Here's how the part is built. I have some questions about the finished solid (model axes, mm). A direction names the side the tool comes from. Round coordinates to 2 decimals unless told otherwise and drop trailing zeros. Order: outer loops, then holes, each group sorted by start corner. A loop starts at its lowest first (then second) coordinate and runs counter-clockwise, first axis right, second up. Notation, with made-up numbers: M 5,34 L 51,34 A8 cw 51,45 Z; hole C 81.25,-26.5 d7. An arc over 180 degrees is marked long. Write item = value, one per line. Start each with the question number.
Item 1: For faces 4 (the face through (1.53, 10.19, 2.95)), 5 (the face through (-0.22, 6.1, -1.71)), which set-ups out of +Z, -Z, +X, -X, +Y, -Y let a thin tool reach every point of the face, with its end or its side?
Item 2: Please list where these lines run through material, in increasing order: L1, parallel to Y at x = -2, z = 0; L2, parallel to Y at x = -1.5, z = 0.25; L3, parallel to X at y = 4.5, z = -1.5.
Item 3: I want a section at A-A, the plane y = 6.5. List the corners of the cut face in (x, z) for me (3 decimals).
Item 4: We'd pull the mould along X, two halves only. Please class faces 1 (the face through (0, 11.1, 0)), 2 (the face through (0.304, 1.141, 0.584)), 3 (the face through (1.35, 9.3, 1.35)): pulls with the +X half, pulls with the -X half, needs draft (parallel to the pull), parting line crosses it, or undercut.
Item 5: I'm going to push flat-ended pins straight in: P1, Ø3, axis at x = -1, y = 5, coming from the -Z side (3 decimals); P2, Ø3, axis at x = -0.5, z = 2, coming from the -Y side; P3, Ø1.5, axis at x = 2.5, y = 10.5, coming from the -Z side. Where does each tip first touch, or does it pass through?
Item 6: I want a section at B-B, the plane y = 2. List the corners of the cut face in (x, z) for me.
```python
from build123d import *

# Parameters (mm, degrees)
CORTAR_EXTRUIR1_START = -1.8
CORTAR_EXTRUIR1_DEPTH = 3


with BuildPart() as part:
    # Croquis1 → Revolución1 (revolve)
    with BuildSketch(Plane.XY):
        with BuildLine():
            Line((0, 0), (0, 11.8))
            ThreePointArc((0, 11.8), (1.722325826, 11.57102319), (3.325, 10.9))
            Line((3.325, 10.9), (3.325, 9.5))
            ThreePointArc((3.325, 9.5), (3.266421356, 9.358578644), (3.125, 9.3))
            Line((3.125, 9.3), (1.725, 9.3))
            Line((1.725, 9.3), (1.725, 2.987787643))
            Line((1.725, 2.987787643), (0, 0))
        make_face()
    revolve(axis=Axis((0, 0, 0), (0, 1, 0)))

    # Croquis2 → Cortar-Extruir1 (cut)
    with BuildSketch(Plane.XZ.offset(-9.3).offset(CORTAR_EXTRUIR1_START)):
        with BuildLine():
            Line((-0.4, 3.2), (-0.4, 0.9))
            ThreePointArc((-0.4, 0.9), (-0.546446609, 0.546446609), (-0.9, 0.4))
            Line((-0.9, 0.4), (-3.2, 0.4))
            Line((-3.2, 0.4), (-3.2, -0.4))
            Line((-3.2, -0.4), (-0.9, -0.4))
            ThreePointArc((-0.9, -0.4), (-0.546446609, -0.546446609), (-0.4, -0.9))
            Line((-0.4, -0.9), (-0.4, -3.2))
            Line((-0.4, -3.2), (0.4, -3.2))
            Line((0.4, -3.2), (0.4, -0.9))
            ThreePointArc((0.4, -0.9), (0.546446609, -0.546446609), (0.9, -0.4))
            Line((0.9, -0.4), (3.2, -0.4))
            Line((3.2, -0.4), (3.2, 0.4))
            Line((3.2, 0.4), (0.9, 0.4))
            ThreePointArc((0.9, 0.4), (0.546446609, 0.546446609), (0.4, 0.9))
            Line((0.4, 0.9), (0.4, 3.2))
            Line((0.4, 3.2), (-0.4, 3.2))
        make_face()
    extrude(amount=-CORTAR_EXTRUIR1_DEPTH, mode=Mode.SUBTRACT)


solid = part.part
```
Filled in:
q1.face_4 = +Y, -Y
q1.face_5 = -Y
q2.L1 = 9.3 to 11.1
q2.L2 = 2.63 to 11.1
q2.L3 = -0.85 to 0.85
q3.outline = C 0,0 d3.45
q4.face_1 = undercut
q4.face_2 = parting line crosses it
q4.face_3 = needs draft
q5.P1 = -1.725
q5.P2 = 0.97
q5.P3 = -2.83
q6.outline = C 0,0 d2.31
